```python
from build123d import *

# Parameters (mm, degrees)
SKETCH3_W           = 160
SKETCH3_H           = 80
SKETCH3_W_2         = 150
SKETCH3_H_2         = 70
BOSS_EXTRUDE2_DEPTH = 5
SKETCH4_W           = 5
SKETCH4_H           = 5
BOSS_EXTRUDE3_DEPTH = 320
BOSS_EXTRUDE4_REACH = 327
SKETCH5_W           = 5
SKETCH5_H           = 80


with BuildPart() as part:
    # Sketch3 → Boss-Extrude2 (new body)
    with BuildSketch(Plane.XY):
        with Locations((80, 40)):
            Rectangle(SKETCH3_W, SKETCH3_H)
        with Locations((80, 40)):
            Rectangle(SKETCH3_W_2, SKETCH3_H_2, mode=Mode.SUBTRACT)
        Polygon((77.5, 75), (77.5, 41.649156988), (77.5, 5), (82.5, 5), (82.5, 41.649156988), (82.5, 75), align=None)
    boss_extrude2 = extrude(amount=BOSS_EXTRUDE2_DEPTH)

    # Sketch4 → Boss-Extrude3 (add)
    with BuildSketch(Plane.XY.offset(5)):
        with Locations((2.5, 2.5)):
            Rectangle(SKETCH4_W, SKETCH4_H)
        with Locations((2.5, 77.5)):
            Rectangle(SKETCH4_W, SKETCH4_H)
        with Locations((157.5, 77.5)):
            Rectangle(SKETCH4_W, SKETCH4_H)
        with Locations((157.5, 2.5)):
            Rectangle(SKETCH4_W, SKETCH4_H)
    extrude(amount=BOSS_EXTRUDE3_DEPTH)

    # Mirror1: Boss-Extrude2 across plane
    add(boss_extrude2.mirror(Plane.XY.offset(165)))

    # Sketch5 → Boss-Extrude4 (add, up to next)
    with BuildSketch(Plane.XY.offset(5), mode=Mode.PRIVATE) as boss_extrude4_sk1:
        with Locations((80, 40)):
            Rectangle(SKETCH5_W, SKETCH5_H)
    boss_extrude4_tool1 = extrude(boss_extrude4_sk1.sketch, amount=BOSS_EXTRUDE4_REACH, mode=Mode.PRIVATE) - part.part
    add(boss_extrude4_tool1.solids().sort_by_distance((80, 40, 5))[0])


solid = part.part
```
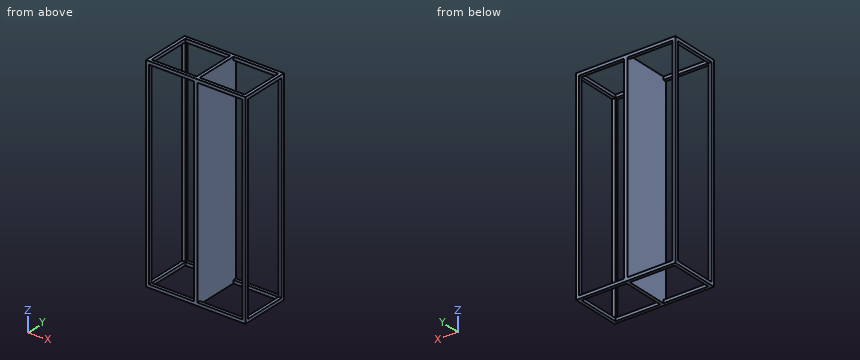
The model under review builds one solid part; all positions refer to its coordinate system, in mm. Round coordinates to 2 decimals unless told otherwise and drop trailing zeros. Loops run counter-clockwise (first coordinate to the right, second up) from the corner with the lowest first, then second, coordinate; pieces in that order, holes last.
1) Clearance check with flat-ended pins moving along their axes: P1, Ø6, axis at y = 30, z = 267, coming from the +X side; P2, Ø1, axis at y = 13, z = 86.5, coming from the -X side. State where each tip first meets the part, or that it passes through.
Values follow:
P1: stops at x = 82.5
P2: stops at x = 77.5
2) Wall thickness on line 1 along X through (y, z) = (75.5, 243.5); line 2 along X through (y, z) = (49, 29.5): over which ranges is each line inside the solid? List them lowest first.
Values follow:
line 1: x = 0 to 5, 77.5 to 82.5, 155 to 160
line 2: x = 77.5 to 82.5
3) Consider section A-A on y = 31.5. State the section outline as (x, z) points, then the cut area to 3 significant figures.
Values follow:
outline: (0, 0) - (5, 0) - (5, 5) - (0, 5) - close; (0, 325) - (5, 325) - (5, 330) - (0, 330) - close; (77.5, 0) - (82.5, 0) - (82.5, 330) - (77.5, 330) - close; (155, 0) - (160, 0) - (160, 5) - (155, 5) - close; (155, 325) - (160, 325) - (160, 330) - (155, 330) - close
area: 1,750 mm2
4) Consider section C-C on z = 260. State the section outline as (x, y) points, then the cut area to 3 significant figures.
Values follow:
outline: (0, 0) - (5, 0) - (5, 5) - (0, 5) - close; (0, 75) - (5, 75) - (5, 80) - (0, 80) - close; (77.5, 0) - (82.5, 0) - (82.5, 80) - (77.5, 80) - close; (155, 0) - (160, 0) - (160, 5) - (155, 5) - close; (155, 75) - (160, 75) - (160, 80) - (155, 80) - close
area: 500 mm2
5) Consider section B-B on x = 58.5. State the section outline as (y, z) points, then the cut area to 3 significant figures.
Values follow:
outline: (0, 0) - (5, 0) - (5, 5) - (0, 5) - close; (0, 325) - (5, 325) - (5, 330) - (0, 330) - close; (75, 0) - (80, 0) - (80, 5) - (75, 5) - close; (75, 325) - (80, 325) - (80, 330) - (75, 330) - close
area: 100 mm2
